Here's how the part is built. I have some questions about the finished solid (model axes, mm). A direction names the side the tool comes from. Round coordinates to 2 decimals unless told otherwise and drop trailing zeros. Loops run counter-clockwise (first coordinate to the right, second up) from the corner with the lowest first, then second, coordinate; pieces in that order, holes last. Notation, with made-up numbers: M 38.5,26.5 L 56.5,26.5 A26 cw 56.5,59.5 Z; hole C 48.5,25.5 d9. An arc over 180 degrees is marked long. Write each question's results on one line, items separated by ' | '. Start each with the question number.
```python
from build123d import *

# Parameters (mm, degrees)
ESBO_O1_R                = 5
RESSALTO_EXTRUS_O1_DEPTH = 5


with BuildPart() as part:
    # Esboço1 → Ressalto-extrusão1 (new body)
    with BuildSketch(Plane.XY):
        with BuildLine():
            Line((-19.446898693, 13.244129565), (-119.446898693, 13.244129565))
            ThreePointArc((-119.446898693, 13.244129565), (-129.446898693, 3.244129565), (-119.446898693, -6.755870435))
            Line((-119.446898693, -6.755870435), (-19.295466425, -6.755870435))
            Line((-19.295466425, -6.755870435), (-19.295466425, -6.754723783))
            ThreePointArc((-19.295466425, -6.754723783), (-9.446898693, 3.244129565), (-19.295466425, 13.242982913))
            ThreePointArc((-19.295466425, 13.242982913), (-19.371180388, 13.243842898), (-19.446898693, 13.244129565))
        make_face()
        with Locations((-119.446898693, 3.244129565)):
            Circle(ESBO_O1_R, mode=Mode.SUBTRACT)
        with BuildLine():
            ThreePointArc((-104.446898693, -1.755870435), (-109.446898693, 3.244129565), (-104.446898693, 8.244129565))
            Line((-104.446898693, 8.244129565), (-34.446898693, 8.244129565))
            ThreePointArc((-34.446898693, 8.244129565), (-29.446898693, 3.244129565), (-34.446898693, -1.755870435))
            Line((-34.446898693, -1.755870435), (-104.446898693, -1.755870435))
        make_face(mode=Mode.SUBTRACT)
        with Locations((-19.446898693, 3.244129565)):
            Circle(ESBO_O1_R, mode=Mode.SUBTRACT)
    extrude(amount=RESSALTO_EXTRUS_O1_DEPTH)


solid = part.part
```
1. Which directions (+Z, -Z, +X, -X, +Y, -Y) give clear straight access to the entire face, cutting with the end or side of a thin tool? Please do faces 4 (the face through (-29.45, 3.35, 2.46)), 5 (the face through (-70, 10, 5)).
2. I want a section at B-B on y = 1.25. List the corners of the cut face in (x, z) for me.
3. I want a section at A-A on x = -118. List the corners of the cut face in (y, z) for me, plus the area to 3 significant figures.
4. I need wall thicknesses on line 1 along Y through (x, z) = (-35.5, 0.2); line 2 along X through (y, z) = (7.75, 1.45); line 3 along X through (y, z) = (3, 3.8). Which ranges of each line are inside material? Lowest first, please.
5. For pin 1 (1.5 mm diameter, centred on y = 2, z = 3.5, fed in from -X), with a flat end and sliding along its axis, tell me the tip position at first contact or that it passes through.
6. If we mould it in two halves opening along X, with no side actions, what happens to faces 1 (the face through (-70, -6.756, 2)), 2 (the face through (-129.444, 3.464, 2.465)), 3 (the face through (-24.442, 3.464, 2.465))? For each: released by +X, released by -X, zero draft, split by the parting line, or undercut.
7. I want a section at C-C on z = 2.8. Count the separate pieces of the cut face and the enclosed holes in it, plus the area to 3 significant figures.
8. I want a section at D-D on y = 11. List the corners of the cut face in (x, z) for me, plus the area to 3 significant figures.
Outcome:
1) face 4: +Z, -Z | face 5: +Z, +X, -X, +Y, -Y
2) outline: M -129.25,0 L -124.03,0 L -124.03,5 L -129.25,5 Z; M -114.86,0 L -109.03,0 L -109.03,5 L -114.86,5 Z; M -29.86,0 L -24.03,0 L -24.03,5 L -29.86,5 Z; M -14.86,0 L -9.65,0 L -9.65,5 L -14.86,5 Z
3) outline: M -6.76,0 L -1.54,0 L -1.54,5 L -6.76,5 Z; M 8.03,0 L 13.24,0 L 13.24,5 L 8.03,5 Z | area: 52.1 mm2
4) line 1: -6.76 to -1.76, 8.24 to 13.24 | line 2: -128.37 to -121.61, -117.28 to -106.61, -32.28 to -21.61, -17.28 to -10.52 | line 3: -129.44 to -124.44, -114.45 to -109.44, -29.45 to -24.44, -14.45 to -9.45
5) pin 1: x = -129.43
6) face 1: zero draft | face 2: released by -X | face 3: undercut
7) separate pieces: 1 | enclosed holes: 3 | area: 1,380 mm2
8) outline: M -125.76,0 L -13.13,0 L -13.13,5 L -125.76,5 Z | area: 563 mm2
